Here's how the part is built. I have some questions about the finished solid (model axes, mm). Face numbers are marked on the shaded views. Round coordinates to 2 decimals unless told otherwise and drop trailing zeros. Loops run counter-clockwise (first coordinate to the right, second up) from the corner with the lowest first, then second, coordinate; pieces in that order, holes last. Notation, with made-up numbers: M 74,56 L 116,56 A32 cw 116,92 Z; hole C -24.75,-11 d11. An arc over 180 degrees is marked long. Use a Markdown table: item, result.
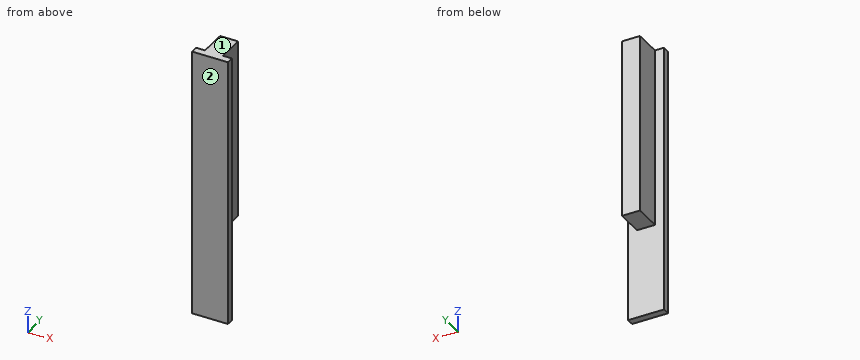
```python
from build123d import *

# Parameters (mm, degrees)
BOSS_EXTRUDE1_DEPTH = 100
BOSS_EXTRUDE2_DEPTH = 50


with BuildPart() as part:
    # Sketch1 → Boss-Extrude1 (new body)
    with BuildSketch(Plane.XY):
        Polygon((10, 4), (5, 4), (-5, 4), (-10, 4), (-10, 0), (10, 0), align=None)
        Polygon((5, 4), (-5, 4), (-5, 9), (-5, 19), (5, 19), (5, 9), align=None)
    extrude(amount=BOSS_EXTRUDE1_DEPTH)

    # Sketch1_3 → Boss-Extrude2 (add)
    with BuildSketch(Plane.XY):
        Polygon((10, 4), (5, 4), (-5, 4), (-10, 4), (-10, 0), (10, 0), align=None)
    extrude(amount=-BOSS_EXTRUDE2_DEPTH)


solid = part.part
```
Q1. I need wall thicknesses on line 1 (Y direction, x = 4.5, z = -42); line 2 (X direction, y = 14.5, z = 79); line 3 (Z direction, x = 2.5, y = 12.5). Which ranges of each line are inside material? Lowest first, please. Write a range as from..to.
Return value:
| item | result |
|---|---|
| line 1 | y = 0..4 |
| line 2 | x = -5..5 |
| line 3 | z = 0..100 |
Q2. Imagine slicing it at B-B, the plane x = 3.75. Please give me the cut outline in (y, z).
Return value:
| item | result |
|---|---|
| outline | M 0,-50 L 4,-50 L 4,0 L 19,0 L 19,100 L 0,100 Z |
Q3. Imagine slicing it at D-D, the plane x = -7. Please give me the cut outline in (y, z).
Return value:
| item | result |
|---|---|
| outline | M 0,-50 L 4,-50 L 4,100 L 0,100 Z |
Q4. Imagine slicing it at A-A, the plane z = 81. Please give me the cut outline in (x, y).
Return value:
| item | result |
|---|---|
| outline | M -10,0 L 10,0 L 10,4 L 5,4 L 5,19 L -5,19 L -5,4 L -10,4 Z |
Q5. Will these pins go through, and if not, where does the flat tip stop? P1, Ø8, axis at y = 15.5, z = 31, coming from the -X side; P2, Ø6, axis at x = -4.5, z = -27, coming from the +Y side; P3, Ø5, axis at x = -1, y = 15, coming from the -Z side.
Return value:
| item | result |
|---|---|
| P1 | stops at x = -5 |
| P2 | stops at y = 4 |
| P3 | stops at z = 0 |
Q6. We'd pull the mould along Z, two halves only. Please class the marked faces 1 and 2: pulls with the +Z half, pulls with the -Z half, needs draft (parallel to the pull), parting line crosses it, or undercut.
Return value:
| item | result |
|---|---|
| face 1 | pulls with the +Z half |
| face 2 | needs draft |
Q7. Imagine slicing it at C-C, the plane y = 15. Please give me the cut outline in (x, z).
Return value:
| item | result |
|---|---|
| outline | M -5,0 L 5,0 L 5,100 L -5,100 Z |
